Model file for the job. Use its own axes, mm. Round coordinates to 2 decimals unless told otherwise and drop trailing zeros. Order: outer loops, then holes, each group sorted by start corner. A loop starts at its lowest first (then second) coordinate and runs counter-clockwise, first axis right, second up. Notation, with made-up numbers: (-19.75, -6.75) -> (28.25, -6.75) arc R26 ccw to (28.25, 13.25) -> close; hole circle Ø1 at (-21, -18.75). An arc over 180 degrees is marked (long way). Use CSV: the item, a comma, the result in double quotes.
Autodesk Inventor part; units mm, degrees
ref_plane "YZ Plane" through (0, 0, 0) normal (1, 0, 0) x (0, 1, 0)
ref_plane "XZ Plane" through (0, 0, 0) normal (0, 1, 0) x (-1, 0, 0)
ref_plane "XY Plane" through (0, 0, 0) normal (0, 0, 1) x (1, 0, 0)
sketch "Sketch1" plane through (0, 0, 0) normal (0, 0, 1) x (1, 0, 0)
  line L0 (-5.4083, 6.8084) -> (-5.4083, 5.8084)
  line L1 (-5.4083, 5.8084) -> (4.5917, 5.8084)
  line L2 (4.5917, 5.8084) -> (4.5917, 9.943)
  arc A0 (4.5917, 9.943) -> (-5.4083, 6.8084) centre (35.0917, -104.875) ccw
  dimension "d24" = 1
extrude "Extrusion1" add sketch "Sketch1" along normal blind 95
sketch "Sketch4" plane through (-5.4083, 5.8084, 0) normal (0, -1, 0) x (1, 0, 0)
  line L0 (0, 95) -> (10, 95)
  line L1 (0, 0) -> (0, 95)
  line L2 (0, 0) -> (10, 0)
  point P0 (5.4083, 0)
  point P1 (5, 12)
  point P2 (5, 83)
  dimension "d25" = 12
  dimension "d26" = 5
  dimension "d27" = 12
  dimension "d28" = 5
hole "Hole2" at (-0.4083, 5.8084, 12) at (-0.4083, 5.8084, 83) direction (0, 1, 0) diameter 4.5 depth 8 tip angle 118
properties part number "podkladka2" material "Ogólne"
Q1. Pin check, flat tips, straight feed: pin 1 (6 mm diameter, centred on x = -0.41, z = 12, fed in from +Y); pin 2 (2.5 mm diameter, centred on x = -0.41, z = 83, fed in from -Y); pin 3 (4 mm diameter, centred on x = -0.5, z = 10, fed in from -Y); pin 4 (1 mm diameter, centred on x = -2, z = 64, fed in from +Y). Stop position of each tip, or through.
From the geometry:
pin 1,"stops at y = 9.39"
pin 2,"passes through"
pin 3,"stops at y = 5.81"
pin 4,"stops at y = 8.15"
Q2. Cut at C-C (z = 37). Give the cut face in (x, y), plus the area to 3 significant figures.
From the geometry:
outline,"(-5.41, 5.81) -> (4.59, 5.81) -> (4.59, 9.94) arc R118.82 ccw to (-5.41, 6.81) -> close"
area,"26.5 mm²"
Q3. Cut at B-B (y = 7.6). Give the cut face in (x, z), plus the area to 3 significant figures.
From the geometry:
outline,"(-3.15, 0) -> (4.59, 0) -> (4.59, 95) -> (-3.15, 95) -> close; hole circle Ø4.5 at (-0.41, 12); hole circle Ø4.5 at (-0.41, 83)"
area,"704 mm²"
Q4. Cut at A-A (z = 12). Give the cut face in (x, y), plus the area to 3 significant figures.
From the geometry:
outline,"(-5.41, 5.81) -> (-2.66, 5.81) -> (-2.66, 7.77) arc R118.82 ccw to (-5.41, 6.81) -> close; (1.84, 5.81) -> (4.59, 5.81) -> (4.59, 9.94) arc R118.82 ccw to (1.84, 9.18) -> close"
area,"14.4 mm²"
Q5. Mould opens along X. For faces 1 (the cylindrical face through (1.788, 7.142, 12.488)), 2 (the flat face through (0, 5.808, 47)), 3 (the flat face through (4.592, 8, 47)) say: +X half, -X half, draft (parallel to the pull), parting line (faces both ways), or undercut.
From the geometry:
face 1,"undercut"
face 2,"draft"
face 3,"+X half"
Q6. Cut at D-D (x = 3.5). Give the cut face in (y, z).
From the geometry:
outline,"(5.81, 0) -> (9.65, 0) -> (9.65, 95) -> (5.81, 95) -> close"
Q7. Probe line 1 along Z through (x, y) = (0.75, 8.7); line 2 along X through (y, z) = (6.65, 83); line 3 along Z through (x, y) = (-2.25, 6). List the from-to ranges inside material, lowest first.
From the geometry:
line 1,"z = 0 to 10.07, 13.93 to 81.07, 84.93 to 95"
line 2,"x = -5.41 to -2.66, 1.84 to 4.59"
line 3,"z = 0 to 10.71, 13.29 to 81.71, 84.29 to 95"
